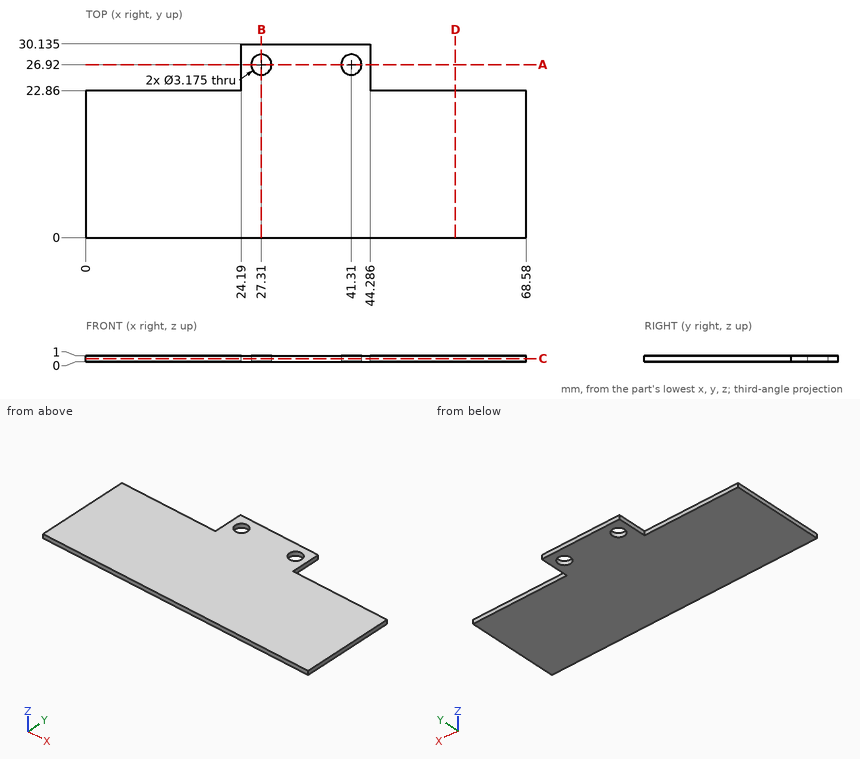
Geometry check sheet. Reference: drawing and pictorial views, mm from the part's lowest x, y, z. Give positions to 0.01 mm unless a question says otherwise; leave off trailing zeros. Write each loop counter-clockwise with the first axis right and the second up, starting at its lowest first coordinate (ties: lowest second). Pieces come first, ordered by that corner, then holes. Notation, with made-up numbers: (89, 25) -> (135, 25) arc R23 ccw to (135, 59) -> close; hole circle Ø10 at (28.25, -31). An arc over 180 degrees is marked (long way). One line per item, written item: value. Start each with the question number.
Item 1: Section check D-D on x = 57.5. Record the cut outline in (y, z).
Item 2: Material ranges on probe 1 along Y at (x, z) = (27.31, 0.6) (1 decimal); probe 2 along Y at (x, z) = (65.5, 0.4); probe 3 along X at (y, z) = (24.5, 0.65) (1 decimal), recorded low to high. Write a range as from..to.
Item 3: Section check A-A on y = 26.92. Record the cut outline in (x, z) (1 decimal).
Item 4: Section check B-B on x = 27.31. Record the cut outline in (y, z) (1 decimal).
Item 5: Gauge pin test, flat ends, axial feed: pin 1 (0.5 mm diameter, centred on y = 25.5, z = 0.5, fed in from +X); pin 2 (3 mm diameter, centred on x = 41.31, y = 26.92, fed in from +Z). Record the tip position at first contact, or that the pin passes through.
Item 6: Section check C-C on z = 0.5. Record the cut outline in (x, y) (1 decimal).
Results list:
1. outline: (0, 0) -> (22.86, 0) -> (22.86, 1) -> (0, 1) -> close
2. probe 1: 0..25.3, 28.5..30.1
2. probe 2: 0..22.86
2. probe 3: 24.2..44.3
3. outline: (24.2, 0) -> (25.7, 0) -> (25.7, 1) -> (24.2, 1) -> close; (28.9, 0) -> (39.7, 0) -> (39.7, 1) -> (28.9, 1) -> close; (42.9, 0) -> (44.3, 0) -> (44.3, 1) -> (42.9, 1) -> close
4. outline: (0, 0) -> (25.3, 0) -> (25.3, 1) -> (0, 1) -> close; (28.5, 0) -> (30.1, 0) -> (30.1, 1) -> (28.5, 1) -> close
5. pin 1: x = 44.29
5. pin 2: through
6. outline: (0, 0) -> (68.6, 0) -> (68.6, 22.9) -> (44.3, 22.9) -> (44.3, 30.1) -> (24.2, 30.1) -> (24.2, 22.9) -> (0, 22.9) -> close; hole circle Ø3.2 at (27.3, 26.9); hole circle Ø3.2 at (41.3, 26.9)
